Read the model definition and answer for the solid it produces. Units are mm, in the model's axes. A direction names the side the tool comes from. Coordinates: 2 decimals unless noted, no trailing zeros. Loops run counter-clockwise (first coordinate to the right, second up) from the corner with the lowest first, then second, coordinate; pieces in that order, holes last. Notation, with made-up numbers: (28, 17.5) -> (59, 17.5) arc R17 ccw to (59, 47.5) -> close; hole circle Ø3 at (29, 84.5). An arc over 180 degrees is marked (long way). Answer in a Markdown table with one row per item.
```python
from build123d import *

# Parameters (mm, degrees)
F0_W     = 34.86
F0_H     = 37.47
F0_R     = 2.8
F0_W_2   = 4.5
F0_H_2   = 6.7
F0_R_2   = 1.6
F1_DEPTH = 2
F2_DEPTH = 6.4


with BuildPart() as f1:
    # F0 (on Top) → F1 (new body)
    with BuildSketch(Plane.XY):
        Rectangle(F0_W, F0_H)
        Polygon((15.03, 16.335), (15.03, -16.335), (-15.03, -16.335), (-15.03, -14.065), (-15.03, 3.565), (-15.03, 16.335), align=None, mode=Mode.SUBTRACT)
        Polygon((-15.03, -16.335), (15.03, -16.335), (15.03, 16.335), (-15.03, 16.335), (-15.03, 3.565), (-8.03, 3.565), (-8.03, -5.735), (-10.53, -5.735), (-10.53, -14.065), (-14.03, -14.065), (-15.03, -14.065), align=None)
        with Locations((3.77, -12.7)):
            Circle(F0_R, mode=Mode.SUBTRACT)
        with Locations((11.22, -8.785)):
            Rectangle(F0_W_2, F0_H_2, mode=Mode.SUBTRACT)
        with Locations((11.22, 0.235)):
            Rectangle(F0_W_2, F0_H_2, mode=Mode.SUBTRACT)
        with Locations((11.22, 9.185)):
            Rectangle(F0_W_2, F0_H_2, mode=Mode.SUBTRACT)
        with Locations((3.77, 12.7)):
            Circle(F0_R, mode=Mode.SUBTRACT)
        Polygon((-15.03, 3.565), (-15.03, -14.065), (-14.03, -14.065), (-10.53, -14.065), (-10.53, -5.735), (-8.03, -5.735), (-8.03, 3.565), align=None)
        with Locations((3.77, 12.7)):
            Circle(F0_R)
        with Locations((3.77, 12.7)):
            Circle(F0_R_2, mode=Mode.SUBTRACT)
        with Locations((3.77, -12.7)):
            Circle(F0_R)
        with Locations((3.77, -12.7)):
            Circle(F0_R_2, mode=Mode.SUBTRACT)
        with Locations((11.22, 9.185)):
            Rectangle(F0_W_2, F0_H_2)
        with Locations((11.22, 0.235)):
            Rectangle(F0_W_2, F0_H_2)
        with Locations((11.22, -8.785)):
            Rectangle(F0_W_2, F0_H_2)
    extrude(amount=F1_DEPTH)

    # F0 (on Top) → F2 (join)
    with BuildSketch(Plane.XY):
        with Locations((3.77, 12.7)):
            Circle(F0_R)
        with Locations((3.77, 12.7)):
            Circle(F0_R_2, mode=Mode.SUBTRACT)
        with Locations((3.77, -12.7)):
            Circle(F0_R)
        with Locations((3.77, -12.7)):
            Circle(F0_R_2, mode=Mode.SUBTRACT)
    extrude(amount=F2_DEPTH)


solid = f1.part
```
1. A cutting plane is placed at A-A on y = -12.7. Give the vertices of the cut face in (x, z).
A:
| item | result |
|---|---|
| outline | (-17.43, 0) -> (2.17, 0) -> (2.17, 6.4) -> (0.97, 6.4) -> (0.97, 2) -> (-17.43, 2) -> close; (5.37, 0) -> (17.43, 0) -> (17.43, 2) -> (6.57, 2) -> (6.57, 6.4) -> (5.37, 6.4) -> close |
2. Find the intervals of material crossed by probe 1 along Y at (x, z) = (3.77, 5); probe 2 along Y at (x, z) = (3.77, 1.75) (3 decimals); probe 3 along Z at (x, y) = (-6, 14), in increasing order.
A:
| item | result |
|---|---|
| probe 1 | y = -15.5 to -14.3, -11.1 to -9.9, 9.9 to 11.1, 14.3 to 15.5 |
| probe 2 | y = -18.735 to -14.3, -11.1 to 11.1, 14.3 to 18.735 |
| probe 3 | z = 0 to 2 |
3. The mould has two halves that part along Y. Classify faces 3 (the flat face through (0, -18.735, 1)), 4 (the flat face through (0, 0, 0)), 5 (the flat face through (0, 18.735, 1)), 6 (the cylindrical face through (3.42, 11.14, 3.16)): pulls with the +Y half, pulls with the -Y half, needs draft (parallel to the pull), parting line crosses it, or undercut.
A:
| item | result |
|---|---|
| face 3 | pulls with the -Y half |
| face 4 | needs draft |
| face 5 | pulls with the +Y half |
| face 6 | undercut |
4. A tool of negligible diameter and unlimited length cuts with its end or side. For faces 1 (the cylindrical face through (3.405, 15.476, 4.169)), 2 (the flat face through (5, 11, 6.4)), from which of +Z, -Z, +X, -X, +Y, -Y can it reach the whole face along a straight path? Write none if from no direction.
A:
| item | result |
|---|---|
| face 1 | +Z |
| face 2 | +Z, +X, -X, +Y, -Y |
5. A cutting plane is placed at C-C on y = 15. Give the vertices of the cut face in (x, z), and give its area (3 significant figures).
A:
| item | result |
|---|---|
| outline | (-17.43, 0) -> (17.43, 0) -> (17.43, 2) -> (5.37, 2) -> (5.37, 6.4) -> (2.17, 6.4) -> (2.17, 2) -> (-17.43, 2) -> close |
| area | 83.8 mm2 |
6. A cutting plane is placed at B-B on x = 3.77. Give the vertices of the cut face in (y, z) (3 decimals), and give its area (3 significant figures).
A:
| item | result |
|---|---|
| outline | (-18.735, 0) -> (-14.3, 0) -> (-14.3, 6.4) -> (-15.5, 6.4) -> (-15.5, 2) -> (-18.735, 2) -> close; (-11.1, 0) -> (11.1, 0) -> (11.1, 6.4) -> (9.9, 6.4) -> (9.9, 2) -> (-9.9, 2) -> (-9.9, 6.4) -> (-11.1, 6.4) -> close; (14.3, 0) -> (18.735, 0) -> (18.735, 2) -> (15.5, 2) -> (15.5, 6.4) -> (14.3, 6.4) -> close |
| area | 83.3 mm2 |
7. Given pin 1 Ø2 at (x, z) = (5, 4.5) entering from -Y; pin 2 Ø4 at (x, y) = (4, -6.5) entering from +Z, each flat-ended and moving along its own axis, determine where each tip first touches the part or whether it passes through.
A:
| item | result |
|---|---|
| pin 1 | stops at y = -15.49 |
| pin 2 | stops at z = 2 |
8. A cutting plane is placed at D-D on x = 8. Give the vertices of the cut face in (y, z) (3 decimals).
A:
| item | result |
|---|---|
| outline | (-18.735, 0) -> (18.735, 0) -> (18.735, 2) -> (-18.735, 2) -> close |
